Can you work these out from the model? Positions are in its coordinate system, mm. A direction names the side the tool comes from. Give positions to 0.01 mm unless a question says otherwise; leave off trailing zeros. Loops run counter-clockwise (first coordinate to the right, second up) from the corner with the lowest first, then second, coordinate; pieces in that order, holes last. Notation, with made-up numbers: (4.25, 24.25) -> (51.25, 24.25) arc R28 cw to (51.25, 50.25) -> close; hole circle Ø8 at (29.5, 71). An arc over 180 degrees is marked (long way). Use CSV: the item, a comma, the result in double quotes.
from build123d import *

# Parameters (mm, degrees)
F1_DEPTH  = 5
F3_DEPTH  = 120
F4_W      = 600
F4_H      = 40
F5_DEPTH  = 5
F7_DEPTH  = 120
F8_W      = 75
F8_H      = 40
F9_DEPTH  = 5
F10_W     = 5
F10_H     = 35
F11_DEPTH = 520
F12_W     = 35
F12_H     = 5
F13_DEPTH = 35
F14_W     = 35
F14_H     = 5
F15_DEPTH = 35


with BuildPart() as f1:
    # F0 (on Top) → F1 (new body)
    with BuildSketch(Plane.XY):
        Polygon((0, -20), (37.5, -20), (37.5, 20), (-37.5, 20), (-37.5, -20), align=None)
    extrude(amount=-F1_DEPTH)

    # F2 (on face) → F3 (join)
    with BuildSketch(Plane.XY):
        Polygon((-32.5, 20), (-37.5, 20), (-37.5, -20), (2.5, -20), (2.5, -15), (-32.5, -15), align=None)
    extrude(amount=F3_DEPTH)

    # F4 (on face) → F5 (join)
    with BuildSketch(Plane.XY.offset(120)):
        with Locations((262.5, 0)):
            Rectangle(F4_W, F4_H)
    extrude(amount=F5_DEPTH)

    # F6 (on face) → F7 (join)
    with BuildSketch(Plane(origin=(0, 0, 120), x_dir=(1, 0, 0), z_dir=(0, 0, -1))):
        Polygon((557.5, -20), (562.5, -20), (562.5, 20), (522.5, 20), (522.5, 15), (557.5, 15), align=None)
    extrude(amount=F7_DEPTH)

    # F8 (on face) → F9 (join)
    with BuildSketch(Plane(origin=(0, 0, 0), x_dir=(1, 0, 0), z_dir=(0, 0, -1))):
        with Locations((525, 0)):
            Rectangle(F8_W, F8_H)
    extrude(amount=F9_DEPTH)

    # F10 (on face) → F11 (join)
    with BuildSketch(Plane.YZ.offset(2.5)):
        with Locations((-17.5, 102.5)):
            Rectangle(F10_W, F10_H)
    extrude(amount=F11_DEPTH)

    # F12 (on face) → F13 (join)
    with BuildSketch(Plane.XY):
        with Locations((20, -17.5)):
            Rectangle(F12_W, F12_H)
    extrude(amount=F13_DEPTH)

    # F14 (on face) → F15 (join)
    with BuildSketch(Plane.XY):
        with Locations((505, -17.5)):
            Rectangle(F14_W, F14_H)
    extrude(amount=F15_DEPTH)


solid = f1.part
(1) If we section it at A-A, the plane z = 30: Write out the boundary of the cut face in (x, y).
Answer sheet:
outline,"(-37.5, -20) -> (37.5, -20) -> (37.5, -15) -> (-32.5, -15) -> (-32.5, 20) -> (-37.5, 20) -> close; (487.5, -20) -> (562.5, -20) -> (562.5, 20) -> (557.5, 20) -> (557.5, -15) -> (487.5, -15) -> close"
(2) If we section it at C-C, the plane x = 148: Write out the boundary of the cut face in (y, z).
Answer sheet:
outline,"(-20, 85) -> (-15, 85) -> (-15, 120) -> (20, 120) -> (20, 125) -> (-20, 125) -> close"
(3) We'd pull the mould along Z, two halves only. Please class faces 4 (the face through (258, -15, 86)), 5 (the face through (-1, 0, -5)), 6 (the face through (37.5, -16, 6)): released by +Z, released by -Z, zero draft, split by the parting line, or undercut.
Answer sheet:
face 4,"undercut"
face 5,"released by -Z"
face 6,"zero draft"
(4) If we section it at D-D, the plane z = 75: Write out the boundary of the cut face in (x, y).
Answer sheet:
outline,"(-37.5, -20) -> (2.5, -20) -> (2.5, -15) -> (-32.5, -15) -> (-32.5, 20) -> (-37.5, 20) -> close; (522.5, -20) -> (562.5, -20) -> (562.5, 20) -> (557.5, 20) -> (557.5, -15) -> (522.5, -15) -> close"
(5) If we section it at B-B, the plane y = -4: Write out the boundary of the cut face in (x, z), then the cut area to 3 significant figures.
Answer sheet:
outline,"(-37.5, -5) -> (37.5, -5) -> (37.5, 0) -> (-32.5, 0) -> (-32.5, 120) -> (557.5, 120) -> (557.5, 0) -> (487.5, 0) -> (487.5, -5) -> (562.5, -5) -> (562.5, 125) -> (-37.5, 125) -> close"
area,"4,950 mm2"
(6) Which directions (+Z, -Z, +X, -X, +Y, -Y) give clear straight access to the entire face, cutting with the end or side of a thin tool? Please do faces 1 (the face through (261, 20, 123)), 2 (the face through (522, 2, 0)), 3 (the face through (487.5, -16, 6)).
Answer sheet:
face 1,"+Z, -Z, +X, -X, +Y"
face 2,"+Y"
face 3,"-Z, +Y, -Y"
(7) Will these pins go through, and if not, where does the flat tip stop? pin 1 Ø4 at (x, y) = (222.5, -18.5) entering from -Z; pin 2 Ø10 at (x, y) = (106, 15) entering from -Z.
Answer sheet:
pin 1,"stops at z = 85"
pin 2,"stops at z = 120"
(8) If I drill on L1, parallel to X at y = -3.5, z = 49; L2, parallel to Z at x = 26, y = 11; L3, parallel to Z at x = 98, y = 3, over which ranges is the centre line in solid material (lowest first)? Write a range as from..to.
Answer sheet:
L1,"x = -37.5..-32.5, 557.5..562.5"
L2,"z = -5..0, 120..125"
L3,"z = 120..125"
